from build123d import *

# Parameters (mm, degrees)
SKETCH_1_R          = 38
SKETCH_1_R_2        = 30
EXTRUDE_1_DEPTH     = 10
SKETCH_2_W          = 8
SKETCH_2_H          = 60
EXTRUDE_2_DEPTH     = 80
SKETCH_3_R          = 4
CUT_EXTRUDE_1_DEPTH = 80
SKETCH_4_W          = 60
SKETCH_4_H          = 40.678120155
CUT_EXTRUDE_2_DEPTH = 97.374270425


with BuildPart() as part:
    # 草图1 → 凸台-拉伸1 (new body)
    with BuildSketch(Plane(origin=(0, 0, 0), x_dir=(1, 0, 0), z_dir=(0, 1, 0))):
        with Locations(Location((0, 0, 0), (0, 0, 270))):
            Circle(SKETCH_1_R)
        with Locations(Location((0, 0, 0), (0, 0, 270))):
            Circle(SKETCH_1_R_2, mode=Mode.SUBTRACT)
    extrude(amount=EXTRUDE_1_DEPTH)

    # 草图2 → 凸台-拉伸2 (add)
    with BuildSketch(Plane.XZ):
        with Locations((-34, 0)):
            Rectangle(SKETCH_2_W, SKETCH_2_H)
        with Locations((34, 0)):
            Rectangle(SKETCH_2_W, SKETCH_2_H)
    extrude(amount=-EXTRUDE_2_DEPTH)

    # 草图3 → 切除-拉伸1 (cut)
    with BuildSketch(Plane(origin=(38, 0, 0), x_dir=(0, 0, -1), z_dir=(1, 0, 0))):
        with Locations((0, 50)):
            Circle(SKETCH_3_R)
        with BuildLine():
            Line((-30, 50), (-30, 88))
            Line((-30, 88), (30, 88))
            Line((30, 88), (30, 50))
            ThreePointArc((30, 50), (0, 80), (-30, 50))
        make_face()
    extrude(amount=-CUT_EXTRUDE_1_DEPTH, mode=Mode.SUBTRACT)

    # 草图4 → 切除-拉伸2 (cut, through all)
    with BuildSketch(Plane.XZ):
        with Locations((0, -20.339060078)):
            Rectangle(SKETCH_4_W, SKETCH_4_H)
    extrude(amount=-CUT_EXTRUDE_2_DEPTH, mode=Mode.SUBTRACT)


solid = part.part
Source: CAD feature listing. Evaluate the final solid. Frame: model axes, mm. A direction names the side the tool comes from. Coordinates: 2 decimals unless noted, no trailing zeros. Loops run counter-clockwise (first coordinate to the right, second up) from the corner with the lowest first, then second, coordinate; pieces in that order, holes last. Notation, with made-up numbers: (37, -12) -> (95, -12) arc R22 ccw to (95, 6) -> close; hole circle Ø6 at (48.5, 87.5). An arc over 180 degrees is marked (long way). Answer in a Markdown table with one row per item. Add a question column.
Q1. Ray query, line 1 along X through (y, z) = (19.5, 26); line 2 along Y through (x, z) = (31, 0); line 3 along X through (y, z) = (8.5, 22). Return the intervals inside material, ascending.
Q2. Section C-C on x = 0. Return the cut outline in (y, z), and give its area (3 significant figures).
Q3. Section A-A on y = 24.5. Return the cut outline in (x, z), and give its area (3 significant figures).
Q4. Reachability of faces 4 (the face through (34.056, 79.993, -0.66)), 5 (the face through (34, 25, 30)), 6 (the face through (0.1, 10, 30.2)), 7 (the face through (-34, 25, 30)) from +Z, -Z, +X, -X, +Y, -Y: full face, straight path, thin tool, end or side. Return the list, or none.
Q5. Section B-B on z = 10.5. Return the cut outline in (x, y).
Q6. Pull-direction query (X, two-part tool) for faces 1 (the face through (30, 39, 0)), 2 (the face through (-33.944, 79.993, -0.66)), 3 (the face through (-38, 39, 0)); classes: pulls with the +X half, pulls with the -X half, needs draft (parallel to the pull), parting line crosses it, or undercut.
Q7. Contact query for flat-ended pins moving along their axis: pin 1 Ø7 at (y, z) = (50, 0) entering from -X; pin 2 Ø2.5 at (x, y) = (33.5, 24) entering from +Z. Output: stop coordinate, or through.
Q8. Section D-D on x = 25. Return the cut outline in (y, z), and give its area (3 significant figures).
Computed values:
| question | item | result |
|---|---|---|
| 1 | line 1 | x = -38 to -30, 30 to 38 |
| 1 | line 2 | y = 0 to 46, 54 to 80 |
| 1 | line 3 | x = -38 to -20.4, 20.4 to 38 |
| 2 | outline | (0, 30) -> (10, 30) -> (10, 38) -> (0, 38) -> close |
| 2 | area | 80.0 mm^2 |
| 3 | outline | (-38, -30) -> (-30, -30) -> (-30, 30) -> (-38, 30) -> close; (30, -30) -> (38, -30) -> (38, 30) -> (30, 30) -> close |
| 3 | area | 960 mm^2 |
| 4 | face 4 | +X, -X, +Y |
| 4 | face 5 | +Z, +X, +Y, -Y |
| 4 | face 6 | +Z, -Z, +Y |
| 4 | face 7 | +Z, -X, +Y, -Y |
| 5 | outline | (-38, 0) -> (-28.1, 0) -> (-28.1, 10) -> (-30, 10) -> (-30, 78.1) -> (-38, 78.1) -> close; (28.1, 0) -> (38, 0) -> (38, 78.1) -> (30, 78.1) -> (30, 10) -> (28.1, 10) -> close |
| 6 | face 1 | undercut |
| 6 | face 2 | needs draft |
| 6 | face 3 | pulls with the -X half |
| 7 | pin 1 | passes through |
| 7 | pin 2 | stops at z = 30 |
| 8 | outline | (0, 16.58) -> (10, 16.58) -> (10, 28.62) -> (0, 28.62) -> close |
| 8 | area | 120 mm^2 |
